from build123d import *

# Parameters (mm, degrees)
BOSS_EXTRUDE1_DEPTH = 6.35
BOSS_EXTRUDE2_REACH = 146.797
BOSS_EXTRUDE4_REACH = 127.921
BOSS_EXTRUDE5_DEPTH = 31.75
SKETCH6_W           = 35.398432863
SKETCH6_H           = 63.441579166
CUT_EXTRUDE3_DEPTH  = 124.542305817
CUT_EXTRUDE2_DEPTH  = 6.35


with BuildPart() as part:
    # Sketch1 → Boss-Extrude1 (new body)
    with BuildSketch(Plane(origin=(0, 0, 0), x_dir=(1, 0, 0), z_dir=(0, 1, 0))):
        Polygon((0, 95.814735378), (-12.7, 95.814735378), (-31.75, 1.834735378), (-68.048716454, -78.671924952), (-49.205184033, -95.703697788), (-12.7, -55.315264622), (0, -55.315264622), align=None)
    extrude(amount=BOSS_EXTRUDE1_DEPTH)

    # Boss-Extrude2: up to this plane
    boss_extrude2_end = Plane(origin=(-31.75, 6.35, -1.834735378), z_dir=(0.9116215886149588, 0, 0.4110305088082135))
    # Sketch3 → Boss-Extrude2 (add, up to the surface)
    with BuildSketch(Plane(origin=(20.527176154, 0, 18.553538338), x_dir=(0.6705422376066268, 0, -0.7418713551455524), z_dir=(0.7418713551455524, 0, 0.6705422376066268)), mode=Mode.PRIVATE) as boss_extrude2_sk1:
        Polygon((-103.993986173, 6.35), (-78.453176795, 24.733648606), (-50.864728594, 38.1), (9.629554025, 38.1), (9.629554025, 6.35), align=None)
    boss_extrude2_tool1 = split(extrude(boss_extrude2_sk1.sketch, amount=-BOSS_EXTRUDE2_REACH, mode=Mode.PRIVATE), bisect_by=boss_extrude2_end, keep=Keep.BOTH, mode=Mode.PRIVATE)
    add(boss_extrude2_tool1.solids().sort_by_distance((-3.940159, 20.681693, 45.623593))[0])

    # Boss-Extrude4: up to this plane
    boss_extrude4_end = Plane(origin=(-12.7, 6.35, -95.814735378), z_dir=(0.9800679771232679, 0, 0.19866242779525697))
    # Sketch4 → Boss-Extrude4 (add, up to the surface)
    with BuildSketch(Plane(origin=(0, 0, -3.158589171), x_dir=(0, 0, 1), z_dir=(-1, 0, 0)), mode=Mode.PRIVATE) as boss_extrude4_sk1:
        Polygon((-92.656146207, 6.35), (1.323853793, 6.35), (1.323853793, 38.1), (-40.992152204, 38.1), (-69.631684908, 23.673473414), align=None)
    boss_extrude4_tool1 = split(extrude(boss_extrude4_sk1.sketch, amount=BOSS_EXTRUDE4_REACH, mode=Mode.PRIVATE), bisect_by=boss_extrude4_end, keep=Keep.BOTH, mode=Mode.PRIVATE)
    add(boss_extrude4_tool1.solids().sort_by_distance((0, 20.310013, -38.759281))[0])

    # Sketch5 → Boss-Extrude5 (add)
    with BuildSketch(Plane(origin=(0, 6.35, 0), x_dir=(1, 0, 0), z_dir=(0, 1, 0))):
        Polygon((0, -41.26429858), (0, -55.315264622), (-12.7, -55.315264622), align=None)
    extrude(amount=BOSS_EXTRUDE5_DEPTH)

    # Sketch6 → Cut-Extrude3 (cut, through all)
    with BuildSketch(Plane(origin=(0, 38.1, 0), x_dir=(1, 0, 0), z_dir=(0, 1, 0))):
        with Locations((17.699216432, -13.706659905)):
            Rectangle(SKETCH6_W, SKETCH6_H)
    extrude(amount=-CUT_EXTRUDE3_DEPTH, mode=Mode.SUBTRACT)

    # Sketch7 → Cut-Extrude2 (cut)
    with BuildSketch(Plane.XZ):
        Polygon((-22.7010489, 66.380177888), (-50.981549283, 40.818778494), (-31.75, -1.834735378), (-17.513793047, -72.066689682), (0, -72.066689682), (0, 55.315264622), (-12.7, 55.315264622), align=None)
    extrude(amount=-CUT_EXTRUDE2_DEPTH, mode=Mode.SUBTRACT)

    # Mirror2: part across plane


with BuildPart() as part_1:
    add(part.part)
    add(part.part.mirror(Plane(origin=(0, 0, 0), x_dir=(0, 0, 1), z_dir=(1, 0, 0))))


solid = part_1.part
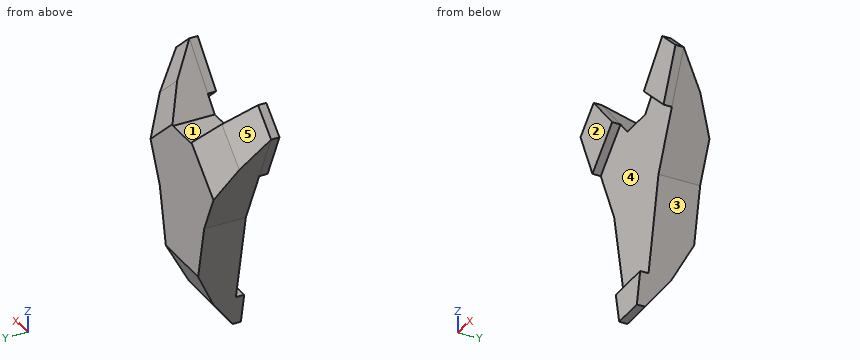
Source: CAD feature listing. Evaluate the final solid. Frame: model axes, mm. Face numbers are marked on the shaded views. A direction names the side the tool comes from. Coordinates: 2 decimals unless noted, no trailing zeros. Order: outer loops, then holes, each group sorted by start corner. A loop starts at its lowest first (then second) coordinate and runs counter-clockwise, first axis right, second up.
Item 1: Cut plane C-C (z = -57). Return loops of the section in (x, y), plus the area to 3 significant figures.
Output values:
outline: (-20.57, 6.35) - (20.57, 6.35) - (20.57, 31.63) - (-20.57, 31.63) - close
area: 1,040 mm2
Item 2: Cut plane D-D (x = -59.5). Return loops of the section in (y, z), plus the area to 3 significant figures.
Output values:
outline: (0, 59.71) - (20.6, 59.71) - (6.35, 86.4) - (0, 86.4) - close
area: 360 mm2
Item 3: Material intervals for line 1 (X direction, y = 5, z = 65); line 2 (Y direction, x = -1, z = 30.5); line 3 (X direction, y = 6, z = 51), sorted ascending.
Output values:
line 1: x = -61.88 to -24.23, 24.23 to 61.88
line 2: y = 6.35 to 38.1
line 3: x = -55.57 to -39.72, 39.72 to 55.57
Item 4: Cut plane B-B (x = -29.5). Return loops of the section in (y, z), plus the area to 3 significant figures.
Output values:
outline: (0, 60.23) - (6.35, 60.23) - (6.35, -12.93) - (38.1, -12.93) - (38.1, 41.9) - (26.6, 73.9) - (0, 73.9) - close
area: 2,660 mm2
Item 5: Pull-direction query (X, two-part tool) for the marked faces 1, 2 and 3; classes: pulls with the +X half, pulls with the -X half, needs draft (parallel to the pull), parting line crosses it, or undercut.
Output values:
face 1: undercut
face 2: needs draft
face 3: pulls with the +X half
Item 6: Cut plane A-A (y = 11). Return loops of the section in (x, z), plus the area to 3 significant figures.
Output values:
outline: (-65.26, 72.49) - (-31.75, -1.83) - (-13.95, -89.63) - (13.95, -89.63) - (31.75, -1.83) - (65.26, 72.49) - (44.87, 90.91) - (12.7, 55.32) - (-12.7, 55.32) - (-44.87, 90.91) - close
area: 11,200 mm2
Item 7: First-contact query: P1, Ø1, axis at x = -2, z = 12.5, coming from the -Y side; P2, Ø12, axis at y = 21, z = 7.5, coming from the -X side; P3, Ø20.5, axis at x = -5.5, y = 15.5, coming from the +Z side. Flat tips, straight axial feed; report the tip coordinate or a pass-through.
Output values:
P1: stops at y = 6.35
P2: stops at x = -38.66
P3: stops at z = 58.69
Item 8: Set-up query: the marked faces 4 and 5. Return all of +Z, -Z, +X, -X, +Y, -Y with unobstructed straight access to the full face (end or side cutting, diameter ignored); none if empty.
Output values:
face 4: -Y
face 5: +Z, -X, +Y
